Here's the drawing with two shaded views (mm, measured from the low corner). I have some questions. A direction names the side the tool comes from. Round coordinates to 2 decimals unless told otherwise and drop trailing zeros. Loops run counter-clockwise (first coordinate to the right, second up) from the corner with the lowest first, then second, coordinate; pieces in that order, holes last. Notation, with made-up numbers: (15, 24.25) -> (52, 24.25) arc R19 cw to (52, 54.25) -> close; hole circle Ø9 at (-1.75, 27.25). An arc over 180 degrees is marked (long way). Use a Markdown table: item, result.
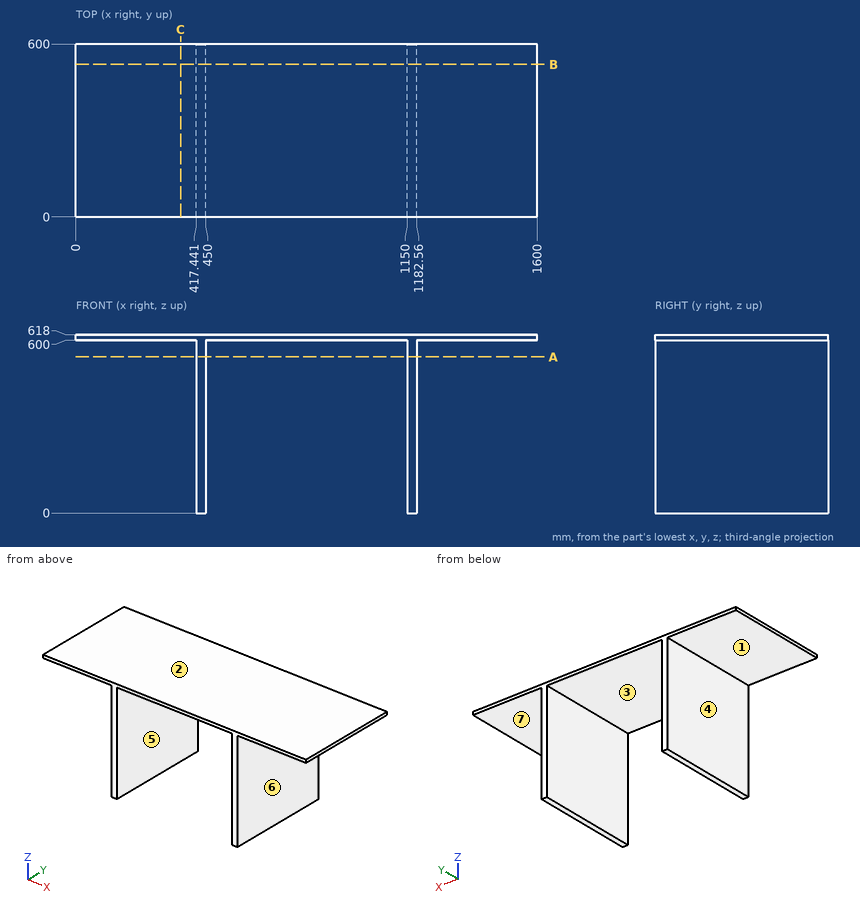
1. If we mould it in two halves opening along X, with no side actions, what happens to the marked faces 4, 5, 6 and 7? For each: +X half, -X half, draft (parallel to the pull), parting line (faces both ways), or undercut.
Answer sheet:
| item | result |
|---|---|
| face 4 | -X half |
| face 5 | undercut |
| face 6 | +X half |
| face 7 | draft |
2. I want a section at C-C (x = 363). Please give me the cut outline in (y, z), plus the area to 3 significant figures.
Answer sheet:
| item | result |
|---|---|
| outline | (0, 600) -> (600, 600) -> (600, 618) -> (0, 618) -> close |
| area | 10,800 mm² |
3. Which directions (+Z, -Z, +X, -X, +Y, -Y) give clear straight access to the entire face, cutting with the end or side of a thin tool? Please do the marked faces 1, 2 and 3.
Answer sheet:
| item | result |
|---|---|
| face 1 | -Z, -X, +Y, -Y |
| face 2 | +Z, +X, -X, +Y, -Y |
| face 3 | -Z, +Y, -Y |
4. Will these pins go through, and if not, where does the flat tip stop? pin 1 Ø2 at (y, z) = (135, 216.5) entering from -X; pin 2 Ø3 at (x, y) = (334.5, 404) entering from -Z.
Answer sheet:
| item | result |
|---|---|
| pin 1 | stops at x = 417.44 |
| pin 2 | stops at z = 600 |
5. I want a section at A-A (z = 542). Please give me the cut outline in (x, y).
Answer sheet:
| item | result |
|---|---|
| outline | (417.44, 0) -> (450, 0) -> (450, 600) -> (417.44, 600) -> close; (1150, 0) -> (1182.56, 0) -> (1182.56, 600) -> (1150, 600) -> close |
6. I need wall thicknesses on line 1 (X direction, y = 246, z = 244.5); line 2 (Z direction, x = 653.5, y = 253.5). Which ranges of each line are inside material? Lowest first, please.
Answer sheet:
| item | result |
|---|---|
| line 1 | x = 417.44 to 450, 1150 to 1182.56 |
| line 2 | z = 600 to 618 |
7. I want a section at B-B (y = 529.5). Please give me the cut outline in (x, z).
Answer sheet:
| item | result |
|---|---|
| outline | (0, 600) -> (417.44, 600) -> (417.44, 0) -> (450, 0) -> (450, 600) -> (1150, 600) -> (1150, 0) -> (1182.56, 0) -> (1182.56, 600) -> (1600, 600) -> (1600, 618) -> (0, 618) -> close |
